from build123d import *

# Parameters (mm, degrees)
SKETCH1_W           = 100.17
SKETCH1_H           = 80.17
BOSS_EXTRUDE1_DEPTH = 3.175
SKETCH2_W           = 6.08
SKETCH2_H           = 6.08
CUT_EXTRUDE2_DEPTH  = 4.175
LPATTERN1_COUNT     = 5
LPATTERN1_PITCH     = 11.0875
SKETCH5_W           = 107.47
SKETCH5_H           = 87.47
SKETCH5_W_2         = 87.47
SKETCH5_H_2         = 67.47
CUT_EXTRUDE4_DEPTH  = 10
SKETCH6_R           = 1.415
CUT_EXTRUDE5_DEPTH  = 10


with BuildPart() as part:
    # Sketch1 → Boss-Extrude1 (new body)
    with BuildSketch(Plane(origin=(0, 0, 0), x_dir=(1, 0, 0), z_dir=(0, 1, 0))):
        Rectangle(SKETCH1_W, SKETCH1_H)
    extrude(amount=BOSS_EXTRUDE1_DEPTH)

    # Sketch2 → Cut-Extrude2 (cut, through all)
    with BuildSketch(Plane(origin=(0, 3.175, 0), x_dir=(1, 0, 0), z_dir=(0, 1, 0))):
        with Locations((-32.175, 22.175)):
            Rectangle(SKETCH2_W, SKETCH2_H)
        with Locations((32.175, 22.175)):
            Rectangle(SKETCH2_W, SKETCH2_H)
    cut_extrude2 = extrude(amount=-CUT_EXTRUDE2_DEPTH, mode=Mode.SUBTRACT)

    # LPattern1: Cut-Extrude2 ×5
    with Locations(*[(0, 0, i * LPATTERN1_PITCH) for i in range(1, LPATTERN1_COUNT)]):
        add(cut_extrude2, mode=Mode.SUBTRACT)

    # Sketch5 → Cut-Extrude4 (cut)
    with BuildSketch(Plane(origin=(0, 3.175, 0), x_dir=(1, 0, 0), z_dir=(0, 1, 0))):
        Rectangle(SKETCH5_W, SKETCH5_H)
        Rectangle(SKETCH5_W_2, SKETCH5_H_2, mode=Mode.SUBTRACT)
    extrude(amount=-CUT_EXTRUDE4_DEPTH, mode=Mode.SUBTRACT)

    # Sketch6 → Cut-Extrude5 (cut)
    with BuildSketch(Plane(origin=(0, 3.175, 0), x_dir=(1, 0, 0), z_dir=(0, 1, 0))):
        with Locations((-40.553019485, 30.553019485)):
            Circle(SKETCH6_R)
        with Locations((-40.553019485, -30.553019485)):
            Circle(SKETCH6_R)
        with Locations((40.553019485, -30.553019485)):
            Circle(SKETCH6_R)
        with Locations((40.553019485, 30.553019485)):
            Circle(SKETCH6_R)
    extrude(amount=-CUT_EXTRUDE5_DEPTH, mode=Mode.SUBTRACT)


solid = part.part
Can you work these out from the model? Positions are in its coordinate system, mm. Coordinates: 2 decimals unless noted, no trailing zeros. Write each loop counter-clockwise with the first axis right and the second up, starting at its lowest first coordinate (ties: lowest second). Pieces come first, ordered by that corner, then holes. Notation, with made-up numbers: (31.5, 14) - (74.5, 14) arc R25 ccw to (74.5, 49) - close; hole circle Ø10 at (-16, -35). An arc over 180 degrees is marked (long way). Return JSON: item names as keys, results as strings. Group by question number.
Item 1: If we section it at B-B (y = 1.1): Count the separate pieces of the cut face and the enclosed holes in it, then the cut area to 3 significant figures.
Item 2: Please list where these lines run through material, in increasing order: probe 1 along X at (y, z) = (2.75, -21) (3 decimals); probe 2 along Z at (x, y) = (-35, 0.7) (1 decimal).
Item 3: I'm going to push a flat-ended pin straight in: pin 1 Ø3.5 at (x, z) = (-40.55, -30.55) entering from -Y. Where does the tip first touch, or does it pass through?
Item 4: If we section it at A-A (z = 0.5): Write out the boundary of the cut face in (x, y) (3 decimals).
Item 5: We'd pull the mould along X, two halves only. Please class faces 1 (the face through (-1, 3.175, 0)), 2 (the face through (-35.215, 2, 22)), 3 (the face through (29.135, 2, -11)): pulls with the +X half, pulls with the -X half, needs draft (parallel to the pull), parting line crosses it, or undercut.
Return value:
{
 "1": {"separate pieces": "1", "enclosed holes": "14", "area": "5,510 mm^2"},
 "2": {"probe 1": "x = -43.735 to -35.215, -29.135 to 29.135, 35.215 to 43.735", "probe 2": "z = -33.7 to -25.2, -19.1 to -14.1, -8 to -3, 3 to 8, 14.1 to 19.1, 25.2 to 33.7"},
 "3": {"pin 1": "stops at y = 0"},
 "4": {"outline": "(-43.735, 0) - (-35.215, 0) - (-35.215, 3.175) - (-43.735, 3.175) - close; (-29.135, 0) - (29.135, 0) - (29.135, 3.175) - (-29.135, 3.175) - close; (35.215, 0) - (43.735, 0) - (43.735, 3.175) - (35.215, 3.175) - close"},
 "5": {"face 1": "needs draft", "face 2": "undercut", "face 3": "undercut"}
}
